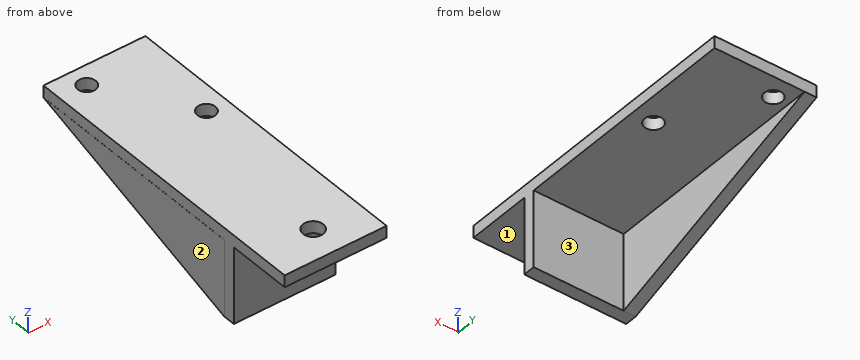
Autodesk Inventor part; units mm, degrees
ref_plane "YZ Plane" through (0, 0, 0) normal (1, 0, 0) x (0, 1, 0)
ref_plane "XZ Plane" through (0, 0, 0) normal (0, 1, 0) x (-1, 0, 0)
ref_plane "XY Plane" through (0, 0, 0) normal (0, 0, 1) x (1, 0, 0)
sketch "Sketch1" plane through (0, 0, 0) normal (0, 1, 0) x (-1, 0, 0)
  line L0 (0, 0) -> (25.4, 0)
  line L1 (25.4, 0) -> (25.4, -20.32)
  line L2 (25.4, -20.32) -> (0, -20.32)
  line L3 (0, -20.32) -> (0, 0)
  dimension "d0" = 25.4
  dimension "d1" = 20.32
extrude "Extrusion1" add sketch "Sketch1" along normal blind 3.1623
sketch "Sketch2" plane through (0, 0, 0) normal (0, -1, 0) x (1, 0, 0)
  line L0 (-25.4, 0) -> (0, 0)
  line L1 (0, 0) -> (0, -20.32)
  line L2 (-25.4, 0) -> (0, 0)
  line L3 (0, 0) -> (0, -3.175)
  line L4 (0, -3.175) -> (-25.4, -3.175)
  line L5 (-25.4, -3.175) -> (-25.4, 0)
  dimension "d4" = 3.175
extrude "Extrusion2" add sketch "Sketch2" along normal blind 17.145
sketch "Sketch3" plane through (0, 3.1623, 0) normal (0, 1, 0) x (1, 0, 0)
  line L0 (-25.4, 0) -> (0, 0)
  line L1 (0, 0) -> (0, 20.32)
  line L2 (-25.4, 0) -> (0, 0)
  line L3 (0, 0) -> (0, 3.175)
  line L4 (0, 3.175) -> (-25.4, 3.175)
  line L5 (-25.4, 3.175) -> (-25.4, 0)
  dimension "d7" = 3.175
extrude "Extrusion3" add sketch "Sketch3" along normal blind 60.96
sketch "Sketch4" plane through (0, 3.1623, -3.175) normal (0, 0, -1) x (-1, 0, 0)
  line L0 (0, 60.96) -> (25.4, 60.96)
  line L1 (25.4, 60.96) -> (19.812, 60.96)
  line L2 (0, 60.96) -> (9.271, 60.96)
  line L3 (0, 0) -> (25.4, 0)
  line L4 (12.7, 0) -> (12.7, 60.96)
  line L5 (12.7, 0) -> (22.733, 0) construction
  line L6 (12.7, 0) -> (2.667, 0) construction
  line L7 (2.667, 0) -> (2.667, 60.96) construction
  line L8 (22.733, 0) -> (22.733, 60.96) construction
  line L9 (25.4, 60.96) -> (0, 60.96) construction
  line L10 (2.667, 60.96) -> (2.667, 21.59) construction
  line L11 (2.667, 21.59) -> (22.733, 21.59) construction
  line L12 (2.667, 60.96) -> (5.588, 60.96) construction
  line L13 (5.588, 60.96) -> (5.588, 21.59) construction
  line L14 (22.733, 60.96) -> (19.812, 60.96) construction
  line L15 (19.812, 60.96) -> (19.812, 21.59) construction
  line L16 (22.733, 60.96) -> (22.733, 55.499) construction
  line L17 (22.733, 55.499) -> (19.812, 55.499) construction
  line L18 (2.667, 21.59) -> (2.667, 33.274) construction
  line L19 (2.667, 33.274) -> (5.588, 33.274) construction
  circle A0 centre (19.812, 55.499) radius 2.3813
  circle A1 centre (5.588, 33.274) radius 2.3813
  point P0 (0, -3.1623)
  dimension "d76" = 10.033
  dimension "d77" = 10.033
  dimension "d78" = 39.37
  dimension "d79" = 2.921
  dimension "d80" = 2.921
  dimension "d81" = 5.461
  dimension "d82" = 11.684
  dimension "d83" = 4.7625
  dimension "d84" = 4.7625
extrude "Extrusion4" cut sketch "Sketch4" against normal blind 63.5
sketch "Sketch7" plane through (0, 0, -3.175) normal (0, 0, -1) x (-1, 0, 0)
  line L0 (25.4, -17.145) -> (0, -17.145)
  line L1 (12.7, -17.145) -> (12.7, -8.5725)
  circle A0 centre (12.7, -8.5725) radius 2.667
  point P0 (0, 0)
  dimension "d23" = 5.334
extrude "Extrusion7" cut sketch "Sketch7" against normal blind 46.0375
move faces "Move1" translate (0, 0, -3.175) faces at (-8.4667, 1.0541, -20.32)
move faces "Move11" translate (-4.7625, 0, 0) faces at (-25.4, 16.7132, -1.0583)
move faces "Move13" translate (1.5875, 0, 0) faces at (-30.1625, 16.7132, -1.0583)
move faces "Move14" translate (1.6002, 0, 0) faces at (-28.575, 16.7132, -1.0583)
sketch "Sketch16" plane through (-30.1625, 0, -23.495) normal (-1, 0, 0) x (0, 0, 1)
  line L0 (0, 3.1623) -> (20.32, 3.1623)
  line L1 (20.32, 3.1623) -> (20.32, 64.1223)
  line L2 (0, 3.1623) -> (20.32, 3.1623)
  line L3 (20.32, 3.1623) -> (20.32, 64.1223)
  line L4 (20.32, 64.1223) -> (0, 3.1623)
  point P0 (23.495, 0)
extrude "Extrusion18" add sketch "Sketch16" against normal blind 6.35
extrude "Extrusion19" cut sketch "Sketch16" against normal blind 3.175
properties part number "SolenoidMount"
Can you work these out from the model? Positions are in its coordinate system, mm. Face numbers are marked on the shaded views. A direction names the side the tool comes from. Give positions to 0.01 mm unless a question says otherwise; leave off trailing zeros. Loops run counter-clockwise (first coordinate to the right, second up) from the corner with the lowest first, then second, coordinate; pieces in that order, holes last. Notation, with made-up numbers: M 57,60.5 L 81,60.5 A29 cw 81,96.5 Z; hole C 3.5,81.25 d6. An arc over 180 degrees is marked long. One line per item, written item: value.
(1) Will these pins go through, and if not, where does the flat tip stop? pin 1 (2 mm diameter, centred on x = -10.5, z = -20, fed in from +Y); pin 2 (1.5 mm diameter, centred on x = -16, z = -19.5, fed in from -Y); pin 3 (8 mm diameter, centred on x = -6, y = 42, fed in from -Z) (3 decimals); pin 4 (1 mm diameter, centred on y = -1, z = -11.5, fed in from +X).
Returned:
pin 1: y = 3.16
pin 2: y = 0
pin 3: z = -3.175
pin 4: through
(2) Suppose I cut it at D-D on y = -7. List the corners of the cut face in (x, z) for me (3 decimals).
Returned:
outline: M -26.975,-3.175 L -14.854,-3.175 L -14.854,0 L -26.975,0 Z; M -10.546,-3.175 L 0,-3.175 L 0,0 L -10.546,0 Z
(3) Suppose I cut it at C-C on x = -1.25. List the corners of the cut face in (y, z) for me (3 decimals).
Returned:
outline: M -17.145,-3.175 L 0,-3.175 L 0,-23.495 L 3.162,-23.495 L 3.162,-3.175 L 64.122,-3.175 L 64.122,0 L -17.145,0 Z
(4) Suppose I cut it at A-A on x = -12.7. List the corners of the cut face in (y, z) for me (1 decimal).
Returned:
outline: M -17.1,-3.2 L -11.2,-3.2 L -11.2,0 L -17.1,0 Z; M -5.9,-3.2 L 0,-3.2 L 0,-23.5 L 3.2,-23.5 L 3.2,-3.2 L 64.1,-3.2 L 64.1,0 L -5.9,0 Z
(5) Suppose I cut it at B-B on z = -2. List the corners of the cut face in (x, y) for me (1 decimal).
Returned:
outline: M -27,-17.1 L 0,-17.1 L 0,64.1 L -27,64.1 Z; hole C -19.8,58.7 d4.8; hole C -12.7,-8.6 d5.3; hole C -5.6,36.4 d4.8
(6) I need wall thicknesses on line 1 (Y direction, x = -12.7, z = -1.2) (1 decimal); line 2 (Z direction, x = -14.75, y = 52.5) (3 decimals); line 3 (X direction, y = 11, z = -18.75). Which ranges of each line are inside material? Lowest first, please.
Returned:
line 1: -17.1 to -11.2, -5.9 to 64.1
line 2: -3.175 to 0
line 3: -26.99 to -23.81
(7) Which directions (+Z, -Z, +X, -X, +Y, -Y) give clear straight access to the entire face, cutting with the end or side of a thin tool? Please do the marked faces 1, 2 and 3.
Returned:
face 1: -Z, +X, -X, -Y
face 2: +Z, -Z, -X, +Y, -Y
face 3: -Z, +X, +Y
